The model under review builds one solid part; all positions refer to its coordinate system, in mm. Give positions to 0.01 mm unless a question says otherwise; leave off trailing zeros. Order: outer loops, then holes, each group sorted by start corner. A loop starts at its lowest first (then second) coordinate and runs counter-clockwise, first axis right, second up. Notation, with made-up numbers: (68.5, -32.75) - (110.5, -32.75) arc R31 ccw to (110.5, 2.25) - close; hole circle Ø5 at (89.5, -21.5). An arc over 180 degrees is marked (long way). Use CSV: the item, a comma, the result in double quotes. Start each with the question number.
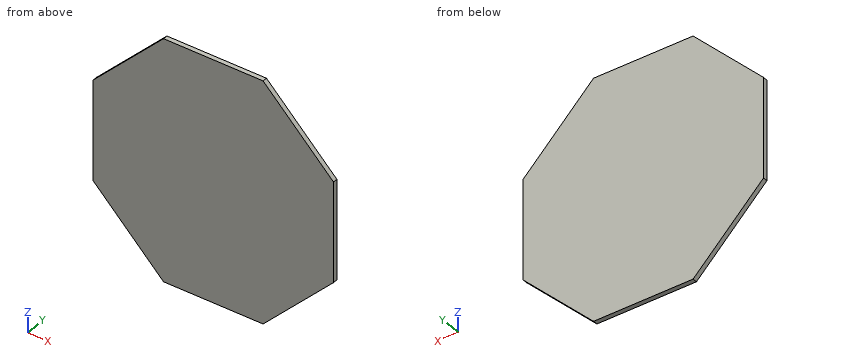
```python
from build123d import *

# Parameters (mm, degrees)
BOSS_EXTRUDE5_DEPTH = 3


with BuildPart() as part:
    # Sketch6 → Boss-Extrude5 (new body)
    with BuildSketch(Plane(origin=(0, 0, 0), x_dir=(1, 0, 0), z_dir=(0, 1, 0))):
        Polygon((78, 32.308657865), (32.308657865, 78), (-32.308657865, 78), (-78, 32.308657865), (-78, -32.308657865), (-32.308657865, -78), (32.308657865, -78), (78, -32.308657865), align=None)
    extrude(amount=-BOSS_EXTRUDE5_DEPTH)


solid = part.part
```
1. Clearance check with flat-ended pins moving along their axes: pin 1 (1.5 mm diameter, centred on y = -1.5, z = 49, fed in from +X); pin 2 (1.5 mm diameter, centred on y = -2.5, z = 47.5, fed in from -X). State where each tip first meets the part, or that it passes through.
2. Consider section C-C (x = 52.5). Give the boundary of the cut face in (y, z), and give its area (3 significant figures).
3. Consider section A-A (y = -1.8). Give the boundary of the cut face in (x, z), and give its area (3 significant figures).
4. Consider section B-B (z = 44.5). Give the boundary of the cut face in (x, y), and give its area (3 significant figures).
5. To check wall thickness, follow L1, parallel to X at y = -1.05, z = -37; L2, parallel to Z at x = -49, y = -0.1; L3, parallel to Z at x = -69, y = -0.4. State the ranges of each line that lie inside material, in increasing order. Write a range as [from, to].
Answers follow:
1,pin 1,"stops at x = 62.06"
1,pin 2,"stops at x = -63.56"
2,outline,"(-3, -57.81) - (0, -57.81) - (0, 57.81) - (-3, 57.81) - close"
2,area,"347 mm^2"
3,outline,"(-78, -32.31) - (-32.31, -78) - (32.31, -78) - (78, -32.31) - (78, 32.31) - (32.31, 78) - (-32.31, 78) - (-78, 32.31) - close"
3,area,"20,200 mm^2"
4,outline,"(-65.81, -3) - (65.81, -3) - (65.81, 0) - (-65.81, 0) - close"
4,area,"395 mm^2"
5,L1,"x = [-73.31, 73.31]"
5,L2,"z = [-61.31, 61.31]"
5,L3,"z = [-41.31, 41.31]"
